from build123d import *

# Parameters (mm, degrees)
F0_R     = 38.1
F0_R_2   = 31.75
F1_DEPTH = 123.825
F2_DEPTH = 9.525
F3_R     = 3.81
F5_DEPTH = 5.08
F6_R     = 2.53999


# Not quite as in the source:
# - a fillet or chamfer that OpenCascade refuses, or shapes differently, is made with other operations: its cross-section is extruded or revolved along the edge and cut away or added
# - a fillet or chamfer is up to 0.001 mm smaller than in the source, because OpenCascade refuses the exact size


with BuildPart() as f1:
    # F0 (on Front) → F1 (new body)
    with BuildSketch(Plane.XZ):
        Circle(F0_R)
        Circle(F0_R_2, mode=Mode.SUBTRACT)
    extrude(amount=F1_DEPTH)

    # F0 (on Front) → F2 (join)
    with BuildSketch(Plane.XZ):
        Circle(F0_R_2)
    extrude(amount=F2_DEPTH)

    # F3
    f3_edges = [f1.edges().sort_by_distance(p)[0] for p in [
        (-38.1, -123.825, 0),
    ]]
    fillet(f3_edges, radius=F3_R)

    # F4: fillet of radius 5.08 on 1 edges, made by hand

    # F4_s1 → F4_t2 (revolve, cut)
    with BuildSketch(Plane.XY):
        with BuildLine():
            ThreePointArc((34.289799962, -123.8253463882), (32.4302345225, -121.9654748362), (31.7496, -119.4250334454))
            Line((31.7496, -119.4250334454), (31.2414634315, -119.4250334454))
            ThreePointArc((31.2414634315, -119.4250334454), (31.2418634315, -121.6250167227), (31.2418634315, -123.825))
            Line((31.2418634315, -123.825), (31.75, -124.3331365685))
            ThreePointArc((31.75, -124.3331365685), (33.019899981, -124.3331365685), (34.0356833896, -124.2653776825))
            Line((34.0356833896, -124.2653776825), (34.289799962, -123.8253463882))
        make_face()
    revolve(axis=Axis((0, -123.825, 0), (0, -1, 0)), mode=Mode.SUBTRACT)

    # F0 (on Front) → F5 (cut)
    with BuildSketch(Plane.XZ):
        Circle(F0_R_2)
    extrude(amount=F5_DEPTH, mode=Mode.SUBTRACT)

    # F6 (radius 2.54 in the source; OpenCascade refuses exactly that, so slightly less here)
    f6_edges = [f1.edges().sort_by_distance(p)[0] for p in [
        (-31.75, -5.08, 0),
        (-31.75, 0, 0),
    ]]
    fillet(f6_edges, radius=F6_R)


solid = f1.part
The model under review builds one solid part; all positions refer to its coordinate system, in mm. A direction names the side the tool comes from. Coordinates: 2 decimals unless noted, no trailing zeros. Loops run counter-clockwise (first coordinate to the right, second up) from the corner with the lowest first, then second, coordinate; pieces in that order, holes last.
(1) Insertion check: P1, Ø6, axis at x = -15, y = -89, coming from the +Z side; P2, Ø12, axis at y = -54, z = -24.5, coming from the -X side; P3, Ø1.5, axis at x = -7, z = 29.5, coming from the +Y side. Each pin has a flat end and moves straight along its axis. Give the tip position at first contact, or say it passes through.
Determined:
P1: stops at z = 36.16
P2: stops at x = -33.31
P3: stops at y = -4.27
(2) Consider section C-C, the plane y = -62. Give the boundary of the cut face in (x, z), plus the area to 3 significant figures.
Determined:
outline: circle Ø76.2 at (0, 0); hole circle Ø63.5 at (0, 0)
area: 1,390 mm2
(3) Draft analysis for pull direction X (two halves, no side actions). For faces 3 (the cylindrical face through (-30.235, -59.167, -23.183)), 4 (the flat face through (-34, 0, 6)), 5 (the flat face through (0, -9.525, 0)), state which applies: +X half, -X half, draft (parallel to the pull), parting line (faces both ways), or undercut.
Determined:
face 3: parting line
face 4: draft
face 5: undercut
(4) Wall thickness on L1, parallel to Z at x = 0, y = -62; L2, parallel to Y at x = 4, z = -7.5 (3 decimals); L3, parallel to X at y = -15.5, z = 28: over which ranges is each line inside the solid? List them lowest first.
Determined:
L1: z = -38.1 to -31.75, 31.75 to 38.1
L2: y = -9.525 to -5.08
L3: x = -25.84 to -14.97, 14.97 to 25.84
(5) Tool access review of faces 1 (the cylindrical face through (-6.883, -63.737, -30.995)), 2 (the flat face through (0, -5.08, 0)): name each direction out of +Z, -Z, +X, -X, +Y, -Y from which nothing blocks a thin tool from reaching the whole face with its end or side.
Determined:
face 1: -Y
face 2: +Y
